Could you check a few things on this model? Use its own coordinates, in mm. Coordinates: 2 decimals unless noted, no trailing zeros. Loops run counter-clockwise (first coordinate to the right, second up) from the corner with the lowest first, then second, coordinate; pieces in that order, holes last. Notation, with made-up numbers: (-12, 78.5) -> (2, 78.5) arc R19 ccw to (2, 85.5) -> close; hole circle Ø3 at (-34.75, 75.5). An arc over 180 degrees is marked (long way). One line per question, with ' | ' between items. Start each with the question number.
(1) Suppose I cut it at B-B (y = 7). Please give me the cut outline in (x, z).
(2) Suppose I cut it at A-A (z = 0). Please give me the cut outline in (x, y).
(3) I'm going to push flat-ended pins straight in: pin 1 Ø5 at (x, y) = (-5.5, 41.5) entering from +Z; pin 2 Ø3.5 at (x, z) = (0, 0) entering from +Y; pin 3 Ø1 at (x, y) = (-2.5, 13) entering from +Z; pin 4 Ø8 at (x, y) = (-4, 24.5) entering from -Z. Where does each tip first touch, or does it pass through?
(4) If I drill on line 1 along X through (y, z) = (0.65, 0); line 2 along Z through (x, y) = (-4.75, 38.5); line 3 along Z through (x, y) = (-6.5, 4.5), over which ranges is the centre line in solid material (lowest first)?
(5) Suppose I cut it at C-C (y = 33.5). Please give me the cut outline in (x, z).
(6) Suppose I cut it at D-D (y = 40). Please give me the cut outline in (x, z).
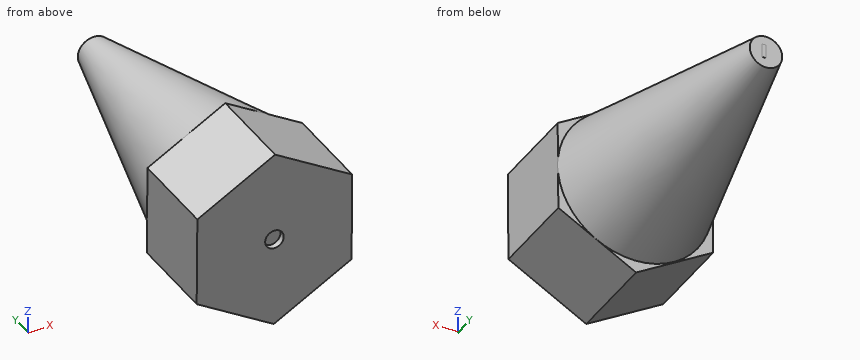
```python
from build123d import *

# Parameters (mm, degrees)
SALIENTE_EXTRUIR1_DEPTH = 15
CROQUIS7_W              = 14.43375673
CROQUIS7_H              = 12.305430405
CORTAR_EXTRUIR1_DEPTH   = 73.231152958
CROQUIS8_R              = 1.5
CORTAR_EXTRUIR2_DEPTH   = 1
CROQUIS10_W             = 0.658671327
CROQUIS10_H             = 2.205507173
SALIENTE_EXTRUIR2_DEPTH = 0.05


with BuildPart() as part:
    # Croquis1 → Saliente-Extruir1 (new body)
    with BuildSketch(Plane(origin=(0, 0, 0), x_dir=(1, 0, 0), z_dir=(0, 1, 0))):
        Polygon((12.555498777, -7.119886502), (12.443751971, 7.313437647), (-0.111746806, 14.433324149), (-12.555498777, 7.119886502), (-12.443751971, -7.313437647), (0.111746806, -14.433324149), align=None)
    extrude(amount=SALIENTE_EXTRUIR1_DEPTH)

    # Croquis6 → Revolución3 (revolve)
    with BuildSketch(Plane.XY, mode=Mode.PRIVATE) as revoluci_n3_sk:
        Polygon((0.111746806, 15), (0.111746806, 65), (12.555498777, 15), align=None)
    revolve(revoluci_n3_sk.sketch.rotate(Axis((0.111746806, 15, 0), (0, 1, 0)), 90), axis=Axis((0.111746806, 15, 0), (0, 1, 0)))

    # Croquis7 → Cortar-Extruir1 (cut, through all)
    with BuildSketch(Plane(origin=(-6.333622792, 0, -10.776605325), x_dir=(-0.8621284260151223, 0, 0.5066898233206265), z_dir=(-0.5066898233206265, 0, -0.8621284260151223))):
        with Locations((0, 60.624376817)):
            Rectangle(CROQUIS7_W, CROQUIS7_H)
    extrude(amount=-CORTAR_EXTRUIR1_DEPTH, mode=Mode.SUBTRACT)

    # Croquis8 → Cortar-Extruir2 (cut)
    with BuildSketch(Plane(origin=(0, 0, 0), x_dir=(-1, 0, 0), z_dir=(0, -1, 0))):
        with Locations(Location((0, 0, 0), (0, 0, 90))):
            Circle(CROQUIS8_R)
    extrude(amount=-CORTAR_EXTRUIR2_DEPTH, mode=Mode.SUBTRACT)

    # Croquis10 → Saliente-Extruir2 (add)
    with BuildSketch(Plane(origin=(0, 54.471661615, 0), x_dir=(1, 0, 0), z_dir=(0, 1, 0))):
        with Locations((0.44108247, -0.051671434)):
            Rectangle(CROQUIS10_W, CROQUIS10_H)
    extrude(amount=SALIENTE_EXTRUIR2_DEPTH)


solid = part.part
```
Checks:
1) outline: (-12.56, -7.12) -> (-0.11, -14.43) -> (12.44, -7.31) -> (12.56, 7.12) -> (0.11, 14.43) -> (-12.44, 7.31) -> close
2) outline: (-12.5, 0) -> (-1.5, 0) -> (-1.5, 1) -> (1.5, 1) -> (1.5, 0) -> (12.5, 0) -> (12.5, 15) -> (12.56, 15) -> (2.73, 54.47) -> (0.77, 54.47) -> (0.77, 54.52) -> (0.11, 54.52) -> (0.11, 54.47) -> (-2.51, 54.47) -> (-12.33, 15) -> (-12.5, 15) -> close
3) pin 1: stops at z = 5.11 | pin 2: stops at y = 54.52 | pin 3: stops at z = 13.24 | pin 4: stops at z = -10.74
4) line 1: x = -12.5 to -1.5, 1.5 to 12.5 | line 2: z = -4.46 to 4.46 | line 3: z = -10.68 to 10.68
5) outline: circle Ø15.68 at (0.11, 0)
6) outline: circle Ø12.44 at (0.11, 0)
